from build123d import *

# Parameters (mm, degrees)
F1_DEPTH      = 6.35
F2_R          = 6.858
F3_DEPTH      = 10.16
F3_DEPTH_BACK = 20.32
F4_R          = 5.08
F5_DEPTH      = 30.48
F6_DEPTH      = 20.32
F7_W          = 3.81
F7_H          = 19.05
F8_DEPTH      = 25.4


with BuildPart() as f1:
    # F0 (on Front) → F1 (new body)
    with BuildSketch(Plane.XZ):
        with BuildLine():
            Line((30.48, 0), (0, 0))
            Line((0, 0), (0, -61.4362284541))
            ThreePointArc((0, -61.4362284541), (14.8767406092, -76.0626361349), (30.48, -62.2138993989))
            Line((30.48, -62.2138993989), (30.48, -59.360794723))
            Line((30.48, -59.360794723), (30.48, 0))
        make_face()
    extrude(amount=F1_DEPTH)

    # F2 (on face) → F3 (join, two sides)
    with BuildSketch(Plane(origin=(0, 0, 0), x_dir=(0, -1, 0), z_dir=(-1, 0, 0))) as f3_sk:
        with Locations((3.175, 6.35)):
            Circle(F2_R)
    extrude(amount=F3_DEPTH)
    extrude(f3_sk.sketch, amount=-F3_DEPTH_BACK)

    # F4 (on face) → F5 (cut)
    with BuildSketch(Plane.YZ.offset(30.48)):
        with Locations((-3.175, 6.35)):
            Circle(F4_R)
    extrude(amount=-F5_DEPTH, mode=Mode.SUBTRACT)

    # F6 (cut): a face of the model
    f6_faces = [f1.faces().sort_by_distance(p)[0] for p in [
        (-10.16, -3.175, 6.35),
    ]]
    extrude(f6_faces, amount=-F6_DEPTH, mode=Mode.SUBTRACT)

    # F7 (on face) → F8 (cut)
    with BuildSketch(Plane.XZ.offset(6.35)):
        with Locations((15.24, -52.242487669)):
            Rectangle(F7_W, F7_H)
    extrude(amount=-F8_DEPTH, mode=Mode.SUBTRACT)


solid = f1.part
Could you check a few things on this model? Use its own coordinates, in mm. A direction names the side the tool comes from. Give positions to 0.01 mm unless a question says otherwise; leave off trailing zeros. Order: outer loops, then holes, each group sorted by start corner. A loop starts at its lowest first (then second) coordinate and runs counter-clockwise, first axis right, second up. Notation, with made-up numbers: (42.25, -20) - (61.25, -20) arc R35 cw to (61.25, 14) - close; hole circle Ø5 at (74, 75). An arc over 180 degrees is marked (long way). One line per question, with ' | ' between items. Start each with the question number.
Item 1: I want a section at B-B on y = -3.75. Write out the boundary of the cut face in (x, z) (3 decimals).
Item 2: I want a section at C-C on x = 5. Write out the boundary of the cut face in (y, z) (3 decimals), then the cut area to 3 significant figures.
Item 3: I need wall thicknesses on probe 1 along Z at (x, y) = (14, -2); probe 2 along X at (y, z) = (-2.25, -49) (3 decimals); probe 3 along Y at (x, z) = (19.5, -34). Which ranges of each line are inside material? Lowest first, please. Write a range as [from, to].
Item 4: I want a section at A-A on z = 6.35. Write out the boundary of the cut face in (x, y) (3 decimals).
Item 5: For faces 5 (the flat face through (15, -6.35, -38)), 6 (the cylindrical face through (5.009, -3.138, -0.508)), 7 (the flat face through (20.32, -4, 12)), 8 (the flat face through (15, -3, -42.717)), which set-ups out of +Z, -Z, +X, -X, +Y, -Y let a thin tool reach every point of the face, with its end or its side?
Item 6: Thinking about a two-plate mould opening in X: for faces 1 (the flat face through (13.335, -3, -52)), 2 (the flat face through (15, 0, -38)), 3 (the cylindrical face through (14.56, -3.13, -76.05)), 4 (the flat face through (17.145, -3, -52)), which applies, pulls with the +X half, pulls with the -X half, needs draft (parallel to the pull), parting line crosses it, or undercut?
Item 7: I want a section at D-D on z = -37. Write out the boundary of the cut face in (x, y), then the cut area to 3 significant figures.
Item 8: I'm going to push flat-ended pins straight in: pin 1 Ø4 at (x, y) = (15, -4) entering from +Z; pin 2 Ø5 at (x, z) = (6.5, -28) entering from +Y; pin 3 Ø10 at (x, z) = (27, -35) entering from -Y; pin 4 Ø3 at (x, y) = (23.5, -0.5) entering from +Z. Where does each tip first touch, or does it pass through?
Verdict:
1) outline: (0, -61.436) arc R15.28 ccw to (30.48, -62.214) - (30.48, 0) - (20.32, 0) - (20.32, 1.303) - (10.16, 1.303) - (10.16, -0.484) - (0, -0.484) - close; (10.16, 11.397) - (20.32, 11.397) - (20.32, 13.184) - (10.16, 13.184) - close; hole (13.335, -61.767) - (17.145, -61.767) - (17.145, -42.717) - (13.335, -42.717) - close
2) outline: (-6.35, -72.105) - (0, -72.105) - (0, 0) - (-0.585, 0) arc R6.858 cw to (-5.765, 0) - (-6.35, 0) - close | area: 456 mm^2
3) probe 1: [-76.02, -61.77], [-42.72, 1.41], [11.29, 13.11] | probe 2: [0, 13.335], [17.145, 30.48] | probe 3: [-6.35, 0]
4) outline: (10.16, -10.033) - (20.32, -10.033) - (20.32, -8.255) - (10.16, -8.255) - close; (10.16, 1.905) - (20.32, 1.905) - (20.32, 3.683) - (10.16, 3.683) - close
5) face 5: -Z, +X, -X, -Y | face 6: +Z, -X | face 7: +Z, +X, +Y, -Y | face 8: +Y, -Y
6) face 1: undercut | face 2: needs draft | face 3: parting line crosses it | face 4: undercut
7) outline: (0, -6.35) - (30.48, -6.35) - (30.48, 0) - (0, 0) - close | area: 194 mm^2
8) pin 1: z = 13.21 | pin 2: y = 0 | pin 3: y = -6.35 | pin 4: z = 0
